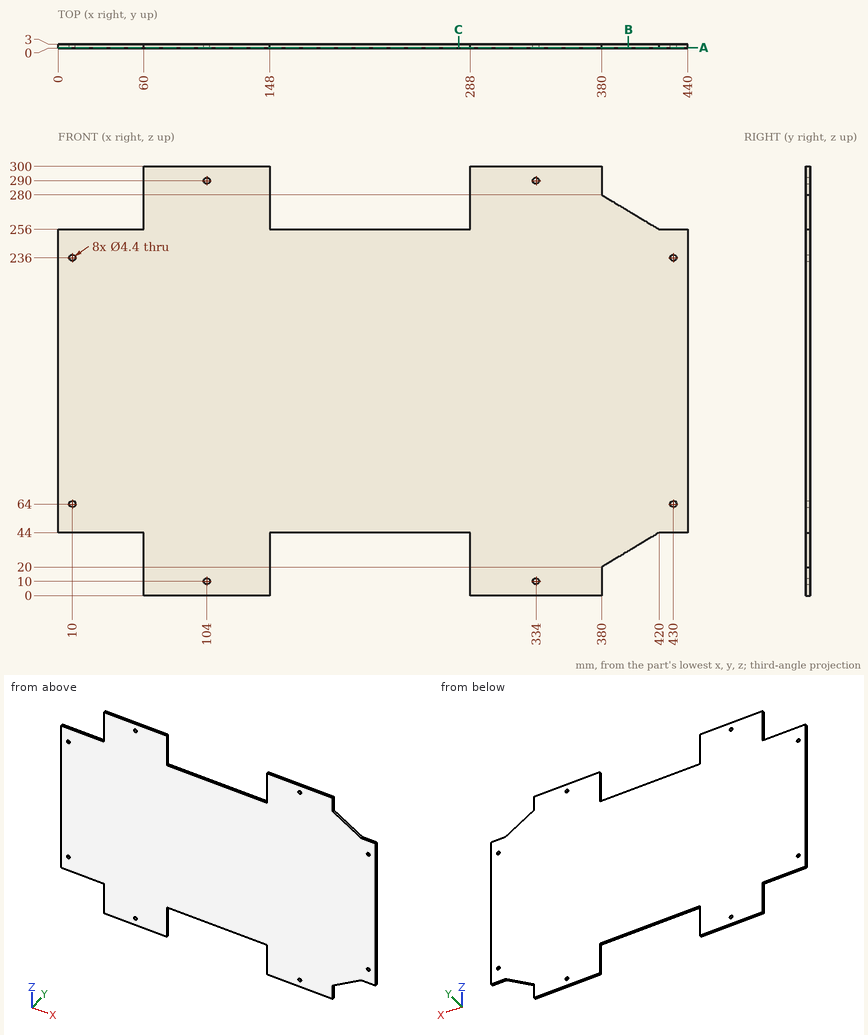
Design review of the part shown in the three views and the two pictorial views. Dimensions are in mm from the part's minimum x, y and z. Coordinates: 2 decimals unless noted, no trailing zeros. Order: outer loops, then holes, each group sorted by start corner. A loop starts at its lowest first (then second) coordinate and runs counter-clockwise, first axis right, second up.
1) Clearance check with flat-ended pins moving along their axes: pin 1 (7 mm diameter, centred on x = 10, z = 236, fed in from -Y); pin 2 (1.5 mm diameter, centred on x = 35.5, y = 1, fed in from +Z); pin 3 (0.9 mm diameter, centred on y = 1, z = 14, fed in from +X); pin 4 (0.9 mm diameter, centred on x = 429, y = 1, fed in from -Z). State where each tip first meets the part, or that it passes through.
2) Take a section at A-A, the plane y = 0.45. State how many separate pieces and enclosed holes the cut face has, and give its area (3 significant figures).
3) Wall thickness on line 1 along X through (y, z) = (0.75, 64); line 2 along Z through (x, y) = (334, 1.9); line 3 along Z through (x, y) = (430, 1.7): over which ranges is each line inside the solid? List them lowest first.
4) Take a section at C-C, the plane x = 280. Give the boundary of the cut face in (y, z).
5) Take a section at B-B, the plane x = 398.5. Give the boundary of the cut face in (y, z), and give its area (3 significant figures).
Returned:
1. pin 1: stops at y = 0
1. pin 2: stops at z = 256
1. pin 3: stops at x = 380
1. pin 4: stops at z = 44
2. separate pieces: 1
2. enclosed holes: 8
2. area: 110,000 mm2
3. line 1: x = 0 to 7.8, 12.2 to 427.8, 432.2 to 440
3. line 2: z = 0 to 7.8, 12.2 to 287.8, 292.2 to 300
3. line 3: z = 44 to 61.8, 66.2 to 233.8, 238.2 to 256
4. outline: (0, 44) - (3, 44) - (3, 256) - (0, 256) - close
5. outline: (0, 31.1) - (3, 31.1) - (3, 268.9) - (0, 268.9) - close
5. area: 713 mm2
